from build123d import *

# Parameters (mm, degrees)
EXTRUDE_1_DEPTH          = 10.5
EXTRUDE_1_DEPTH_BACK     = 6
FILLET_1_R               = 2
CUT_EXTRUDE_1_DEPTH      = 51.301816014
CUT_EXTRUDE_1_DEPTH_BACK = 51.301816014
SKETCH_2_R               = 5
CUT_EXTRUDE_2_DEPTH      = 2.25
EXTRUDE_3_DEPTH          = 9.401473572


with BuildPart() as part:
    # Эскиз1 → Бобышка-Вытянуть1 (new, two sides: drawn at the far end of the back side and taken through both)
    with BuildSketch(Plane(origin=(0, 0, 0), x_dir=(1, 0, 0), z_dir=(0, 1, 0)).offset(-EXTRUDE_1_DEPTH_BACK)):
        with BuildLine():
            Line((-26.485281374, 38.5), (-26.485281374, 55.65945007))
            Line((-26.485281374, 55.65945007), (-39.508260541, 53.069018453))
            ThreePointArc((-39.508260541, 53.069018453), (-49.589786713, 47.94606891), (-55.52997461, 38.323389984))
            Line((-55.52997461, 38.323389984), (-58.010710812, 29.67203472))
            Line((-58.010710812, 29.67203472), (-55.847871996, 29.05185067))
            Line((-55.847871996, 29.05185067), (-52.002825213, 27.949301246))
            Line((-52.002825213, 27.949301246), (-48.695176943, 39.484441598))
            Line((-48.695176943, 39.484441598), (-39.657900512, 36.893044281))
            Line((-39.657900512, 36.893044281), (-42.965548782, 25.35790393))
            Line((-42.965548782, 25.35790393), (-39.120501998, 24.255354507))
            Line((-39.120501998, 24.255354507), (-36.777584474, 32.426078922))
            add(Edge.make_bspline(
                [(-36.777584474, 32.426078922), (-35.035915631, 38.5), (-29.380741372, 38.5)],
                knots=[0, 0, 0, 1, 1, 1], degree=2))
            Line((-29.380741372, 38.5), (-26.485281374, 38.5))
        make_face()
    extrude(amount=EXTRUDE_1_DEPTH + EXTRUDE_1_DEPTH_BACK)

    # Скругление1
    fillet_1_edges = [part.edges().sort_by_distance(p)[0] for p in [
        (-34.198352133, 10.5, -36.862455815),
        (-27.933011373, 10.5, -38.5),
        (-32.996770958, 10.5, -54.364234261),
        (-49.589786713, 10.5, -47.94606891),
        (-37.949043236, -6, -28.340716715),
        (-56.770342711, -6, -33.997712352),
        (-56.770342711, 10.5, -33.997712352),
        (-49.589786713, -6, -47.94606891),
        (-32.996770958, -6, -54.364234261),
        (-27.933011373, -6, -38.5),
        (-34.198352133, -6, -36.862455815),
        (-37.949043236, 10.5, -28.340716715),
    ]]
    fillet(fillet_1_edges, radius=FILLET_1_R)

    # Эскиз2 → Вырез-Вытянуть1 (cut, two sides: drawn at the far end of the back side and taken through both)
    with BuildSketch(Plane(origin=(-55.457297641, 0, -15.902124205), x_dir=(-0.27563735581600457, 0, 0.9612616959386041), z_dir=(-0.9612616959386041, 0, -0.27563735581600457)).offset(-CUT_EXTRUDE_1_DEPTH_BACK)):
        with BuildLine():
            Line((-18.53267148, -6), (-12.53267148, -6))
            Line((-12.53267148, -6), (-12.53267148, 0))
            ThreePointArc((-12.53267148, 0), (-14.290030793, -4.242640687), (-18.53267148, -6))
        make_face()
        with Locations((-18.53267148, 0)):
            Circle(SKETCH_2_R)
    extrude(amount=CUT_EXTRUDE_1_DEPTH + CUT_EXTRUDE_1_DEPTH_BACK, mode=Mode.SUBTRACT)

    # Эскиз4 → Вырез-Вытянуть2 (cut)
    with BuildSketch(Plane(origin=(-61.46518324, 0, -17.624857679), x_dir=(-0.2756373558160068, 0, 0.9612616959386036), z_dir=(-0.9612616959386036, 0, -0.2756373558160068))):
        with BuildLine():
            Line((-16.03267148, 6), (-12.53267148, 6))
            Line((-12.53267148, 6), (-12.53267148, 2.5))
            Line((-12.53267148, 2.5), (-12.53267148, -6))
            Line((-12.53267148, -6), (-21.032671479, -6))
            Line((-21.032671479, -6), (-24.53267148, -6))
            Line((-24.53267148, -6), (-24.53267148, -2.499999999))
            ThreePointArc((-24.53267148, -2.499999999), (-23.128865557, 4.596194078), (-16.03267148, 6))
        make_face()
    extrude(amount=-CUT_EXTRUDE_2_DEPTH, mode=Mode.SUBTRACT)

    # Эскиз5 → Бобышка-Вытянуть3 (add)
    with BuildSketch(Plane(origin=(-46.42002121, 0, -13.310726889), x_dir=(-0.2756373558157037, 0, 0.9612616959386904), z_dir=(-0.9612616959386904, 0, -0.2756373558157037))):
        with BuildLine():
            Line((-24.53267148, 10.5), (-24.53267148, -6))
            Line((-24.53267148, -6), (-18.53267148, -6))
            ThreePointArc((-18.53267148, -6), (-14.290030793, -4.242640687), (-12.53267148, 0))
            Line((-12.53267148, 0), (-12.53267148, 10.5))
            Line((-12.53267148, 10.5), (-24.53267148, 10.5))
        make_face()
    extrude(amount=EXTRUDE_3_DEPTH)


solid = part.part
Geometry check sheet. Reference: the model listing, model coordinates, mm. A direction names the side the tool comes from. Round coordinates to 2 decimals unless told otherwise and drop trailing zeros. Write each question's results on one line, items separated by ' | '. Start each with the question number.
1. Set-up check for faces 1 (the face through (-27.91, -5.4, -39.07)), 2 (the face through (-53.53, -4.27, -40.87)), 3 (the face through (-50.33, 0.07, -33.78)), 4 (the face through (-27.91, 9.9, -39.07)), 5 (the face through (-28, 2, -38.5)): record each of +Z, -Z, +X, -X, +Y, -Y from which the full face is reachable in a straight line by a thin tool's end or side.
2. Draft check along Z on faces 6 (the face through (-32.977, 9.899, -53.787)), 7 (the face through (-41.292, 0.07, -31.193)), 8 (the face through (-26.485, 2, -47)), 9 (the face through (-38.226, 4.94, -27.376)). Enter one of: pulls with the +Z half, pulls with the -Z half, needs draft (parallel to the pull), parting line crosses it, or undercut.
3. Go/stop test with flat-tipped pins: P1, Ø3, axis at x = -28, y = -1, coming from the +Z side; P2, Ø5, axis at y = 6.5, z = -49, coming from the -X side; P3, Ø1.6, axis at x = -56, z = -31, coming from the -Y side. Record where each tip stops, or that it passes through.
4. Material ranges on L1, parallel to Y at x = -41, z = -27; L2, parallel to Y at x = -50, z = -36; L3, parallel to Z at x = -29, y = -1, recorded low to high. Write a range as from..to.
Resolved:
1) face 1: +Z, +X, -Y | face 2: -X, -Y | face 3: none | face 4: +Z, +X, +Y | face 5: +Z, +X, +Y, -Y
2) face 6: pulls with the -Z half | face 7: undercut | face 8: needs draft | face 9: pulls with the +Z half
3) P1: z = -38.5 | P2: x = -51.02 | P3: y = -4.68
4) L1: -4.58..-3.15, 3.15..10.5 | L2: -6..-4.44, 4.44..10.5 | L3: -55.16..-38.5
